Source: CAD feature listing. Evaluate the final solid. Frame: model axes, mm. A direction names the side the tool comes from. Give positions to 0.01 mm unless a question says otherwise; leave off trailing zeros. Order: outer loops, then holes, each group sorted by start corner. A loop starts at its lowest first (then second) coordinate and runs counter-clockwise, first axis right, second up. Notation, with made-up numbers: M 18,38 L 48,38 A24 ccw 48,73 Z; hole C -34.75,6.5 d8. An arc over 180 degrees is marked long. Answer in a Markdown table with one row per item. Add a question column.
(1) Section query C-C, the plane y = 26. Return loops of the section in (x, z), plus the area to 3 significant figures.
(2) Section query D-D, the plane z = 25. Return loops of the section in (x, y), plus the area to 3 significant figures.
(3) Pin query (flat end, axial travel): P1, Ø1, axis at x = 4, z = 34.5, coming from the -Y side; P2, Ø3, axis at x = 1, z = 40.5, coming from the -Y side; P3, Ø1.5, axis at x = 4.5, z = 97.5, coming from the -Y side. Return the tip coordinate at first contact, or that it passes through.
(4) Set-up query: faces 5 (the face through (2.55, -36.75, 13.56)), 6 (the face through (2.553, -114.363, 130.686)). Return all of +Z, -Z, +X, -X, +Y, -Y with unobstructed straight access to the full face (end or side cutting, diameter ignored); none if empty.
(5) Material intervals for line 1 along Y through (x, z) = (4.35, 127.5); line 2 along Z through (x, y) = (2.1, 70.5); line 3 along Z through (x, y) = (3.9, 59), sorted ascending.
(6) Section query A-A, the plane z = -44. Return loops of the section in (x, y), plus the area to 3 significant figures.
(7) Section query B-B, the plane x = 1.05. Count the separate pieces of the cut face and the enclosed holes in it, plus the area to 3 significant figures.
(8) Mould query, pull axis Y, two halves, no side actions, for faces 1 (the face through (0, -22, 27)), 2 (the face through (2.553, -100.763, 124.463)), 3 (the face through (2.55, 78.36, -95.92)), 4 (the face through (2.553, -8.145, 41.792)). Classes: pulls with the +Y half, pulls with the -Y half, needs draft (parallel to the pull), parting line crosses it, or undercut.
from build123d import *

# Parameters (mm, degrees)
SKETCH1_R           = 7.7375
SKETCH1_R_2         = 1.6
BOSS_EXTRUDE1_DEPTH = 5.1784


with BuildPart() as part:
    # Sketch1 → Boss-Extrude1 (new body)
    with BuildSketch(Plane(origin=(0, 0, 0), x_dir=(0, 0, -1), z_dir=(1, 0, 0))):
        with BuildLine():
            Line((-148.619647966, -94.78818035), (68.068798078, 80.959130728))
            ThreePointArc((68.068798078, 80.959130728), (96.200393571, 78.024282343), (93.265545186, 49.89268685))
            Line((93.265545186, 49.89268685), (-123.422900858, -125.854624227))
            ThreePointArc((-123.422900858, -125.854624227), (-151.554496351, -122.919775842), (-148.619647966, -94.78818035))
        make_face()
        with Locations((80.667171632, 65.425908789)):
            Circle(SKETCH1_R, mode=Mode.SUBTRACT)
        with Locations((45.71742227, 37.079568293)):
            Circle(SKETCH1_R, mode=Mode.SUBTRACT)
        with Locations((-141.564832381, -124.796172236)):
            Circle(SKETCH1_R_2, mode=Mode.SUBTRACT)
        with Locations((-151.328571886, -112.757925234)):
            Circle(SKETCH1_R_2, mode=Mode.SUBTRACT)
        with Locations((-145.785013917, -98.283155286)):
            Circle(SKETCH1_R_2, mode=Mode.SUBTRACT)
        with Locations((-130.477716443, -95.84663234)):
            Circle(SKETCH1_R_2, mode=Mode.SUBTRACT)
        with Locations((-120.713976939, -107.884879343)):
            Circle(SKETCH1_R_2, mode=Mode.SUBTRACT)
        with Locations((-126.257534908, -122.359649291)):
            Circle(SKETCH1_R_2, mode=Mode.SUBTRACT)
        with BuildLine():
            Line((-125.325183683, -110.015390658), (-136.19843904, -118.834252146))
            ThreePointArc((-136.19843904, -118.834252146), (-145.341207576, -117.880426421), (-144.387381851, -108.737657886))
            Line((-144.387381851, -108.737657886), (-133.514126493, -99.918796398))
            ThreePointArc((-133.514126493, -99.918796398), (-124.371357958, -100.872622123), (-125.325183683, -110.015390658))
        make_face(mode=Mode.SUBTRACT)
    extrude(amount=BOSS_EXTRUDE1_DEPTH)


solid = part.part
Values follow:
| question | item | result |
|---|---|---|
| 1 | outline | M 0,-63.81 L 5.18,-63.81 L 5.18,-0.31 L 0,-0.31 Z |
| 1 | area | 329 mm² |
| 2 | outline | M 0,-46.03 L 5.18,-46.03 L 5.18,5.47 L 0,5.47 Z |
| 2 | area | 267 mm² |
| 3 | P1 | stops at y = -54.14 |
| 3 | P2 | stops at y = -59.82 |
| 3 | P3 | stops at y = -105.44 |
| 4 | face 5 | -Z, +X, -X, -Y |
| 4 | face 6 | +X, -X |
| 5 | line 1 | y = -128.42 to -123.37, -121.35 to -111.78, -98.76 to -77.66 |
| 5 | line 2 | z = -100.01 to -86.51, -74.83 to -55.17 |
| 5 | line 3 | z = -99.61 to -84.98, -76.36 to -40.99 |
| 6 | outline | M 0,9.94 L 5.18,9.94 L 5.18,29.54 L 0,29.54 Z; M 0,44.62 L 5.18,44.62 L 5.18,61.44 L 0,61.44 Z |
| 6 | area | 189 mm² |
| 7 | separate pieces | 1 |
| 7 | enclosed holes | 9 |
| 7 | area | 11,700 mm² |
| 8 | face 1 | needs draft |
| 8 | face 2 | undercut |
| 8 | face 3 | parting line crosses it |
| 8 | face 4 | pulls with the +Y half |
